Autodesk Inventor part; units mm, degrees
ref_plane "YZ Plane" through (0, 0, 0) normal (1, 0, 0) x (0, 1, 0)
ref_plane "XZ Plane" through (0, 0, 0) normal (0, 1, 0) x (-1, 0, 0)
ref_plane "XY Plane" through (0, 0, 0) normal (0, 0, 1) x (1, 0, 0)
sketch "Skizze1" plane through (0, 0, 0) normal (0, 0, 1) x (1, 0, 0)
  line L0 (-2.5, -20) -> (2.5, -20)
  line L1 (2.5, -20) -> (2.5, 20)
  line L2 (2.5, 20) -> (-2.5, 20)
  line L3 (-2.5, 20) -> (-2.5, -20)
  line L4 (-2.5, -20) -> (2.5, 20) construction
  line L5 (2.5, -20) -> (-2.5, 20) construction
  point P0 (0, 0)
  dimension "d0" = 5
  dimension "d1" = 40
extrude "Extrusion1" add sketch "Skizze1" along normal blind 380
sketch "Skizze2" plane through (2.5, -20, 0) normal (1, 0, 0) x (0, 0, -1)
  line L0 (0, 0) -> (0, 40)
  line L1 (0, 40) -> (-380, 40)
  line L2 (-380, 0) -> (-380, 40)
  line L3 (0, 0) -> (-380, 0)
  point P0 (0, 20)
  point P1 (-190, 20)
  point P2 (0, 20)
  dimension "d4" = 380
  dimension "d5" = 190
hole "Bohrung1" at (2.5, 0, 190) direction (-1, 0, 0) diameter 6 end through all
properties part number "Querstrebe_camera" material "Holz (Eiche)"
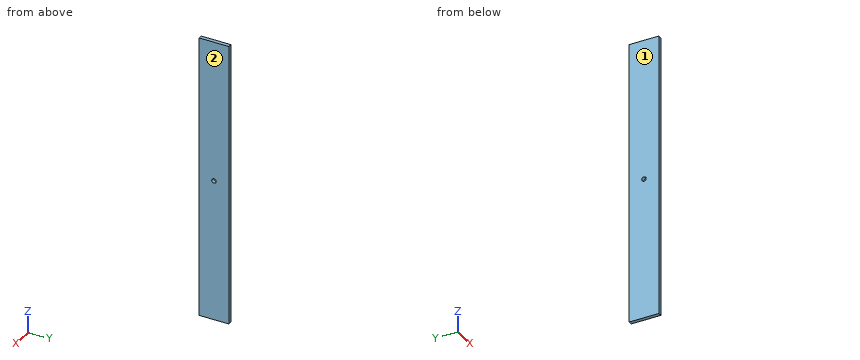
Can you work these out from the model? Positions are in its coordinate system, mm. Face numbers are marked on the shaded views. Coordinates: 2 decimals unless noted, no trailing zeros. Return JSON: item names as keys, results as strings. Group by question number.
Item 1: Please list where these lines run through material, in increasing order: probe 1 along Y at (x, z) = (0.3, 190); probe 2 along Z at (x, y) = (0.3, 0); probe 3 along Z at (x, y) = (-1.3, -2).
Item 2: I'm going to push a flat-ended pin straight in: pin 1 Ø7 at (y, z) = (0, 190) entering from -X. Where does the tip first touch, or does it pass through?
Item 3: We'd pull the mould along X, two halves only. Please class the marked faces 1 and 2: pulls with the +X half, pulls with the -X half, needs draft (parallel to the pull), parting line crosses it, or undercut.
Return value:
{
 "1": {"probe 1": "y = -20 to -3, 3 to 20", "probe 2": "z = 0 to 187, 193 to 380", "probe 3": "z = 0 to 187.76, 192.24 to 380"},
 "2": {"pin 1": "stops at x = -2.5"},
 "3": {"face 1": "pulls with the -X half", "face 2": "pulls with the +X half"}
}
